Part model, mm, in its own coordinate system. A direction names the side the tool comes from. Round coordinates to 2 decimals unless told otherwise and drop trailing zeros. Loops run counter-clockwise (first coordinate to the right, second up) from the corner with the lowest first, then second, coordinate; pieces in that order, holes last.
from build123d import *

# Parameters (mm, degrees)
CUT_EXTRUDE1_DEPTH  = 10
CIRPATTERN1_COUNT   = 4
SKETCH3_R           = 11
CUT_EXTRUDE2_DEPTH  = 82.111035008
CIRPATTERN2_COUNT   = 3
SKETCH5_R           = 2.5
BOSS_EXTRUDE1_DEPTH = 13
CIRPATTERN3_COUNT   = 3


with BuildPart() as part:
    # Sketch1 → Revolve2 (revolve)
    with BuildSketch(Plane.XY, mode=Mode.PRIVATE) as revolve2_sk:
        Polygon((16, 0), (16, 13), (45, 13), (45, 36), (55, 36), (55, 0), align=None)
    revolve(revolve2_sk.sketch.rotate(Axis((0, 0, 0), (0, 1, 0)), 90), axis=Axis((0, 0, 0), (0, 1, 0)))

    # Sketch2 → Cut-Extrude1 (cut)
    with BuildSketch(Plane(origin=(0, 36, 0), x_dir=(1, 0, 0), z_dir=(0, 1, 0))):
        with BuildLine():
            Line((44.72135955, 5), (54.772255751, 5))
            ThreePointArc((54.772255751, 5), (55, 0), (54.772255751, -5))
            Line((54.772255751, -5), (44.72135955, -5))
            ThreePointArc((44.72135955, -5), (45, 0), (44.72135955, 5))
        make_face()
    cut_extrude1 = extrude(amount=-CUT_EXTRUDE1_DEPTH, mode=Mode.SUBTRACT)

    # CirPattern1: Cut-Extrude1 ×4 about axis
    cirpattern1_axis = Axis((0, 0, 0), (0, 1, 0))
    for i in range(1, CIRPATTERN1_COUNT):
        add(cut_extrude1.rotate(cirpattern1_axis, i * 360 / CIRPATTERN1_COUNT), mode=Mode.SUBTRACT)

    # Sketch3 → Cut-Extrude2 (cut, through all)
    with BuildSketch(Plane(origin=(0, 13, 0), x_dir=(1, 0, 0), z_dir=(0, 1, 0))):
        with Locations(Location((0, -32, 0), (0, 0, 270))):
            Circle(SKETCH3_R)
    cut_extrude2 = extrude(amount=-CUT_EXTRUDE2_DEPTH, mode=Mode.SUBTRACT)

    # CirPattern2: Cut-Extrude2 ×3 about axis
    cirpattern2_axis = Axis((0, 0, 0), (0, 1, 0))
    for i in range(1, CIRPATTERN2_COUNT):
        add(cut_extrude2.rotate(cirpattern2_axis, i * 360 / CIRPATTERN2_COUNT), mode=Mode.SUBTRACT)

    # Sketch5 → Boss-Extrude1 (add)
    with BuildSketch(Plane.XZ):
        with BuildLine():
            Line((-6.5, 54.614558499), (-3.419696086, 68.745438584))
            ThreePointArc((-3.419696086, 68.745438584), (0, 71.5), (3.419696086, 68.745438584))
            Line((3.419696086, 68.745438584), (6.5, 54.614558499))
            ThreePointArc((6.5, 54.614558499), (0, 55), (-6.5, 54.614558499))
        make_face()
        with Locations(Location((0, 68, 0), (0, 0, 270))):
            Circle(SKETCH5_R, mode=Mode.SUBTRACT)
    boss_extrude1 = extrude(amount=-BOSS_EXTRUDE1_DEPTH)

    # CirPattern3: Boss-Extrude1 ×3 about axis
    cirpattern3_axis = Axis((0, 0, 0), (0, 1, 0))
    for i in range(1, CIRPATTERN3_COUNT):
        add(boss_extrude1.rotate(cirpattern3_axis, i * 360 / CIRPATTERN3_COUNT))


solid = part.part
1) Slice it at C-C, the plane x = -20. Give the cut face in (y, z), then the cut area to 3 significant figures.
Values:
outline: (0, -51.23) - (36, -51.23) - (36, -40.31) - (13, -40.31) - (13, -23.84) - (0, -23.84) - close; (0, -8.16) - (13, -8.16) - (13, 40.31) - (36, 40.31) - (36, 51.23) - (0, 51.23) - close
area: 1,630 mm2
2) Wall check: line 1 along Z through (x, y) = (-0.5, 2); line 2 along X through (y, z) = (4, 0); line 3 along X through (y, z) = (20, -23). Give the ranges that are in metal, low to high.
Values:
line 1: z = -55 to -15.99, 15.99 to 21.01, 42.99 to 65.55, 70.45 to 71.46
line 2: x = -55 to -16, 16 to 55
line 3: x = -49.96 to -38.68, 38.68 to 49.96
3) Slice it at B-B, the plane z = 0. Give the cut face in (x, y).
Values:
outline: (-55, 0) - (-16, 0) - (-16, 13) - (-45, 13) - (-45, 26) - (-55, 26) - close; (16, 0) - (55, 0) - (55, 26) - (45, 26) - (45, 13) - (16, 13) - close
4) Drop flat-ended pins along their axis: pin 1 Ø3 at (x, y) = (50, 33) entering from -Z; pin 2 Ø3 at (y, z) = (11, -14.5) entering from -X; pin 3 Ø8 at (x, z) = (17.5, -26.5) entering from -Y; pin 4 Ø6 at (x, z) = (58.89, -34) entering from +Y. Give the stop position or say it passes through.
Values:
pin 1: stops at z = -25.94
pin 2: stops at x = -53.44
pin 3: stops at y = 0
pin 4: stops at y = 13
5) Mould opens along X. For faces 4 (the face through (-55.97, 6.41, -26.61)), 5 (the face through (-5, 31, 50)), 6 (the face through (50, 31, 5)) say: released by +X, released by -X, zero draft, split by the parting line, or undercut.
Values:
face 4: released by -X
face 5: undercut
face 6: zero draft
6) Slice it at D-D, the plane z = -39. Give the cut face in (x, y), then the cut area to 3 significant figures.
Values:
outline: (-38.78, 0) - (38.78, 0) - (38.78, 36) - (22.45, 36) - (22.45, 13) - (-22.45, 13) - (-22.45, 36) - (-38.78, 36) - close
area: 1,760 mm2
7) Slice it at A-A, the plane y = 30.5. Give the cut face in (x, z).
Values:
outline: (-54.77, -5) arc R55 ccw to (-5, -54.77) - (-5, -44.72) arc R45 cw to (-44.72, -5) - close; (-54.77, 5) - (-44.72, 5) arc R45 cw to (-5, 44.72) - (-5, 54.77) arc R55 ccw to start; (5, -54.77) arc R55 ccw to (54.77, -5) - (44.72, -5) arc R45 cw to (5, -44.72) - close; (5, 44.72) arc R45 cw to (44.72, 5) - (54.77, 5) arc R55 ccw to (5, 54.77) - close
8) Tool access for faces 1 (the face through (17.235, 24.661, -41.569)), 2 (the face through (-50.84, 6.409, -35.105)), 3 (the face through (-50, 31, -5)): list every direction of +Z, -Z, +X, -X, +Y, -Y with a clear straight run to the whole face (end or side of a thin tool).
Values:
face 1: +Y
face 2: -Z, +Y, -Y
face 3: +X, -X, +Y
